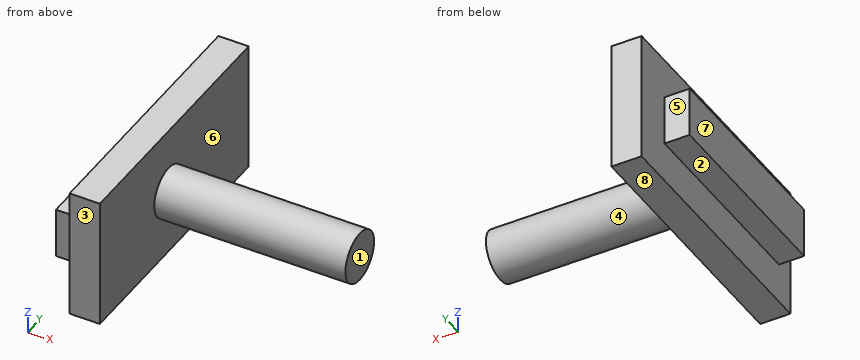
Autodesk Inventor part; units mm, degrees
ref_plane "YZ Plane" through (0, 0, 0) normal (1, 0, 0) x (0, 1, 0)
ref_plane "XZ Plane" through (0, 0, 0) normal (0, 1, 0) x (-1, 0, 0)
ref_plane "XY Plane" through (0, 0, 0) normal (0, 0, 1) x (1, 0, 0)
sketch "Sketch1" plane through (0, 0, 0) normal (0, 0, 1) x (1, 0, 0)
  line L0 (0, 0) -> (3, 0)
  line L1 (3, 0) -> (3, 26)
  line L2 (3, 26) -> (0, 26)
  line L3 (0, 26) -> (0, 0)
  line L4 (-2.5, 22) -> (0, 22)
  line L5 (0, 22) -> (0, 2)
  line L6 (0, 2) -> (-2.5, 2)
  line L7 (-2.5, 2) -> (-2.5, 22)
  point P0 (-1.25, 2)
  point P1 (0, 22)
  dimension "d0" = 2.5
  dimension "d1" = 20
  dimension "d2" = 26
  dimension "d3" = 3
  dimension "d4" = 2
extrude "Extrusion1" add sketch "Sketch1" along normal blind 5
sketch "Sketch2" plane through (3, 0, 0) normal (1, 0, 0) x (0, 0, -1)
  circle A0 centre (-2.5, 12) radius 2.5
  line L0 (0, 0) -> (0, 26)
  line L1 (0, 26) -> (-5, 26)
  point P0 (-2.5, 26)
  dimension "d7" = 14
extrude "Extrusion2" add sketch "Sketch2" along normal blind 19
sketch "Sketch3" plane through (3, 26, 5) normal (1, 0, 0) x (0, 0, -1)
  line L0 (5, -26) -> (9, -26)
  line L1 (9, -26) -> (9, 0)
  line L2 (9, 0) -> (5, 0)
  line L3 (5, 0) -> (5, -26)
  line L4 (0, -26) -> (-4, -26)
  line L5 (-4, -26) -> (-4, 0)
  line L6 (-4, 0) -> (0, 0)
  line L7 (0, 0) -> (0, -26)
  dimension "d10" = 4
  dimension "d11" = 4
extrude "Extrusion3" add sketch "Sketch3" against normal blind 3
properties part number "contact_axis"
Can you work these out from the model? Positions are in its coordinate system, mm. Face numbers are marked on the shaded views. A direction names the side the tool comes from. Round coordinates to 2 decimals unless told otherwise and drop trailing zeros. Loops run counter-clockwise (first coordinate to the right, second up) from the corner with the lowest first, then second, coordinate; pieces in that order, holes last. Notation, with made-up numbers: (-8, -23) -> (-1, -23) arc R14 ccw to (-1, -11) -> close; hole circle Ø6 at (-15, 83). An arc over 180 degrees is marked (long way). One line per item, written item: value. Start each with the question number.
1. If we section it at A-A, the plane y = 15: Write out the boundary of the cut face in (x, z).
2. If we section it at B-B, the plane z = 2.5: Write out the boundary of the cut face in (x, y), then the cut area to 3 significant figures.
3. If we section it at C-C, the plane x = 15.25: Write out the boundary of the cut face in (y, z).
4. If I drill on probe 1 along X at (y, z) = (18.25, 3.5); probe 2 along Z at (x, y) = (-1.25, 12.75); probe 3 along X at (y, z) = (5, -2.5), over which ranges is the centre line in solid material (lowest first)?
5. For pin 1 (4 mm diameter, centred on y = 22.5, z = 1.5, fed in from +X); pin 2 (3 mm diameter, centred on x = 18.5, z = 7, fed in from +Y); pin 3 (3 mm diameter, centred on x = 5, z = 3.5, fed in from -Y); pin 4 (1.2 mm diameter, centred on x = -1.5, z = 1.5, fed in from +Y), each with a flat end and sliding along its axis, tell me the tip position at first contact or that it passes through.
6. If we mould it in two halves opening along X, with no side actions, what happens to the marked faces 6, 7 and 8? For each: pulls with the +X half, pulls with the -X half, needs draft (parallel to the pull), parting line crosses it, or undercut.
7. For the marked faces 1, 2, 3, 4 and 5, which set-ups out of +Z, -Z, +X, -X, +Y, -Y let a thin tool reach every point of the face, with its end or its side?
8. If we section it at D-D, the plane y = 12: Write out the boundary of the cut face in (x, z), then the cut area to 4 significant figures.
Calculated:
1. outline: (-2.5, 0) -> (0, 0) -> (0, -4) -> (3, -4) -> (3, 9) -> (0, 9) -> (0, 5) -> (-2.5, 5) -> close
2. outline: (-2.5, 2) -> (0, 2) -> (0, 0) -> (3, 0) -> (3, 9.5) -> (22, 9.5) -> (22, 14.5) -> (3, 14.5) -> (3, 26) -> (0, 26) -> (0, 22) -> (-2.5, 22) -> close
2. area: 223 mm²
3. outline: circle Ø5 at (12, 2.5)
4. probe 1: x = -2.5 to 3
4. probe 2: z = 0 to 5
4. probe 3: x = 0 to 3
5. pin 1: stops at x = 3
5. pin 2: passes through
5. pin 3: stops at y = 9.5
5. pin 4: stops at y = 22
6. face 6: pulls with the +X half
6. face 7: pulls with the -X half
6. face 8: needs draft
7. face 1: +Z, -Z, +X, +Y, -Y
7. face 2: -Z, -X, +Y, -Y
7. face 3: +Z, -Z, +X, -X, -Y
7. face 4: +X
7. face 5: +Z, -Z, -X, +Y
8. outline: (-2.5, 0) -> (0, 0) -> (0, -4) -> (3, -4) -> (3, 0) -> (22, 0) -> (22, 5) -> (3, 5) -> (3, 9) -> (0, 9) -> (0, 5) -> (-2.5, 5) -> close
8. area: 146.5 mm²
